Can you work these out from the model? Positions are in its coordinate system, mm. A direction names the side the tool comes from. Coordinates: 2 decimals unless noted, no trailing zeros. Write each loop counter-clockwise with the first axis right and the second up, starting at its lowest first coordinate (ties: lowest second). Pieces come first, ordered by that corner, then holes. Notation, with made-up numbers: (-11, 8) - (41, 8) arc R21 ccw to (41, 12) - close; hole circle Ø5 at (46, 84). An arc over 180 degrees is marked (long way). Use one line per item in the form item = value. Start each with the question number.
(1) For pin 1 Ø18 at (x, y) = (0, 0) entering from -Z, with a flat end and sliding along its axis, tell me the tip position at first contact or that it passes through.
(2) Thinking about a two-plate mould opening in X: for faces 3 (the face through (96.99, 97.15, 15.21)), 4 (the face through (80, -70, 15)), 5 (the face through (-1, -100, 15)), which applies, pulls with the +X half, pulls with the -X half, needs draft (parallel to the pull), parting line crosses it, or undercut?
(3) If we section it at C-C on z = 10.75: Please give me the cut outline in (x, y).
(4) On a 3-axis mill with a long thin cutter (end or side, diameter ignored), from which of +Z, -Z, +X, -X, +Y, -Y can I reach the whole of each face in a straight line? I mean faces 1 (the face through (-0.806, 59.995, 14.79)), 2 (the face through (96.99, -97.15, 15.21)). Say none if no direction works.
(5) If we section it at B-B on y = -70: Please give me the cut outline in (x, z), then the cut area to 3 significant figures.
(6) If we section it at D-D on x = 36.5: Please give me the cut outline in (y, z), then the cut area to 3 significant figures.
(7) If I drill on probe 1 along Y at (x, z) = (5.5, 21); probe 2 along Y at (x, z) = (38, 26); probe 3 along Y at (x, z) = (70.5, 23.75), over which ranges is the centre line in solid material (lowest first)? Write a range as from..to.
(8) If we section it at A-A on x = 0: Please give me the cut outline in (y, z).
```python
from build123d import *

# Parameters (mm, degrees)
SKETCH1_W           = 200
SKETCH1_H           = 200
SKETCH1_R           = 10
BOSS_EXTRUDE1_DEPTH = 30
FILLET1_R           = 10


with BuildPart() as part:
    # Sketch1 → Boss-Extrude1 (new body)
    with BuildSketch(Plane.XY):
        Rectangle(SKETCH1_W, SKETCH1_H)
        Circle(SKETCH1_R, mode=Mode.SUBTRACT)
        with BuildLine():
            Line((70, -80), (-70, -80))
            ThreePointArc((-70, -80), (-80, -70), (-70, -60))
            Line((-70, -60), (70, -60))
            ThreePointArc((70, -60), (80, -70), (70, -80))
        make_face(mode=Mode.SUBTRACT)
        with BuildLine():
            ThreePointArc((65.532163543, 45.886114908), (0, 80), (-65.532163543, 45.886114908))
            ThreePointArc((-65.532163543, 45.886114908), (-63.076407464, 31.958830102), (-49.149122657, 34.414586181))
            ThreePointArc((-49.149122657, 34.414586181), (0, 60), (49.149122657, 34.414586181))
            ThreePointArc((49.149122657, 34.414586181), (63.076407464, 31.958830102), (65.532163543, 45.886114908))
        make_face(mode=Mode.SUBTRACT)
    extrude(amount=BOSS_EXTRUDE1_DEPTH)

    # Fillet1
    fillet1_edges = [part.edges().sort_by_distance(p)[0] for p in [
        (-100, 100, 15),
        (100, 100, 15),
        (100, -100, 15),
        (-100, -100, 15),
    ]]
    fillet(fillet1_edges, radius=FILLET1_R)


solid = part.part
```
Reported:
q1.pin_1 = through
q2.face_3 = pulls with the +X half
q2.face_4 = undercut
q2.face_5 = needs draft
q3.outline = (-100, -90) arc R10 ccw to (-90, -100) - (90, -100) arc R10 ccw to (100, -90) - (100, 90) arc R10 ccw to (90, 100) - (-90, 100) arc R10 ccw to (-100, 90) - close; hole (-70, -80) - (70, -80) arc R10 ccw to (70, -60) - (-70, -60) arc R10 ccw to start; hole (-65.53, 45.89) arc R10 ccw to (-49.15, 34.41) arc R60 cw to (49.15, 34.41) arc R10 ccw to (65.53, 45.89) arc R80 ccw to start; hole circle Ø20 at (0, 0)
q4.face_1 = +Z, -Z
q4.face_2 = +Z, -Z, +X, -Y
q5.outline = (-100, 0) - (-80, 0) - (-80, 30) - (-100, 30) - close; (80, 0) - (100, 0) - (100, 30) - (80, 30) - close
q5.area = 1,200 mm2
q6.outline = (-100, 0) - (-80, 0) - (-80, 30) - (-100, 30) - close; (-60, 0) - (47.62, 0) - (47.62, 30) - (-60, 30) - close; (71.19, 0) - (100, 0) - (100, 30) - (71.19, 30) - close
q6.area = 4,690 mm2
q7.probe_1 = -100..-80, -60..-8.35, 8.35..59.75, 79.81..100
q7.probe_2 = -100..-80, -60..46.43, 70.4..100
q7.probe_3 = -100..-79.99, -60.01..100
q8.outline = (-100, 0) - (-80, 0) - (-80, 30) - (-100, 30) - close; (-60, 0) - (-10, 0) - (-10, 30) - (-60, 30) - close; (10, 0) - (60, 0) - (60, 30) - (10, 30) - close; (80, 0) - (100, 0) - (100, 30) - (80, 30) - close
